from build123d import *

# Parameters (mm, degrees)
SKETCH1_W               = 292
SKETCH1_H               = 117
SKETCH1_R               = 1.75
BOSS_EXTRUDE1_DEPTH     = 4.5
SKETCH1_3_R             = 1.75
CUT_EXTRUDE1_DEPTH      = 4.5
MIRROR3_COPY_1_SKETCH_R = 1.75
MIRROR3_COPY_1_DEPTH    = 4.5
SKETCH2_W               = 35
SKETCH2_H               = 140
BOSS_EXTRUDE2_DEPTH     = 30
CHAMFER1_SIZE           = 10
CHAMFER1_SIZE2          = 15
CHAMFER2_SIZE           = 15
CHAMFER2_SIZE2          = 10


with BuildPart() as part:
    # Sketch1 → Boss-Extrude1 (new body)
    with BuildSketch(Plane.XY):
        Rectangle(SKETCH1_W, SKETCH1_H)
        with Locations((-90, 44)):
            Circle(SKETCH1_R, mode=Mode.SUBTRACT)
        with Locations((-90, 44)):
            Circle(SKETCH1_R)
    extrude(amount=BOSS_EXTRUDE1_DEPTH)

    # Sketch1_3 → Cut-Extrude1 (cut)
    with BuildSketch(Plane.XY):
        with Locations((-90, 44)):
            Circle(SKETCH1_3_R)
    cut_extrude1 = extrude(amount=CUT_EXTRUDE1_DEPTH, mode=Mode.SUBTRACT)

    # Mirror2: Cut-Extrude1 across plane
    add(cut_extrude1.mirror(Plane.ZX), mode=Mode.SUBTRACT)

    # Mirror3: Cut-Extrude1 across plane
    add(cut_extrude1.mirror(Plane(origin=(0, 0, 0), x_dir=(0, 0, 1), z_dir=(1, 0, 0))), mode=Mode.SUBTRACT)

    # Mirror3 copy 1 sketch → Mirror3 copy 1 (cut)
    with BuildSketch(Plane(origin=(0, 0, 0), x_dir=(-1, 0, 0), z_dir=(0, 0, 1))):
        with Locations((-90, 44)):
            Circle(MIRROR3_COPY_1_SKETCH_R)
    extrude(amount=MIRROR3_COPY_1_DEPTH, mode=Mode.SUBTRACT)

    # Sketch2 → Boss-Extrude2 (add)
    with BuildSketch(Plane(origin=(0, 0, 0), x_dir=(-1, 0, 0), z_dir=(0, 0, -1))):
        with Locations((-128.5, 11.5)):
            Rectangle(SKETCH2_W, SKETCH2_H)
    boss_extrude2 = extrude(amount=-BOSS_EXTRUDE2_DEPTH)

    # Chamfer1
    chamfer1_edges = [part.edges().sort_by_distance(p)[0] for p in [
        (128.5, 81.5, 0),
    ]]
    chamfer1_side = [part.faces().sort_by_distance(p)[0] for p in [
        (128.5, 81.5, 15),
    ]]
    chamfer(chamfer1_edges, length=CHAMFER1_SIZE, length2=CHAMFER1_SIZE2, reference=chamfer1_side[0])

    # Mirror5: Boss-Extrude2 across plane
    add(boss_extrude2.mirror(Plane(origin=(0, 0, 0), x_dir=(0, 0, 1), z_dir=(1, 0, 0))))

    # Chamfer2
    chamfer2_edges = [part.edges().sort_by_distance(p)[0] for p in [
        (-128.5, 81.5, 0),
    ]]
    chamfer2_side = [part.faces().sort_by_distance(p)[0] for p in [
        (-1.915975925, 2.0973848, 0),
    ]]
    chamfer(chamfer2_edges, length=CHAMFER2_SIZE, length2=CHAMFER2_SIZE2, reference=chamfer2_side[0])


solid = part.part
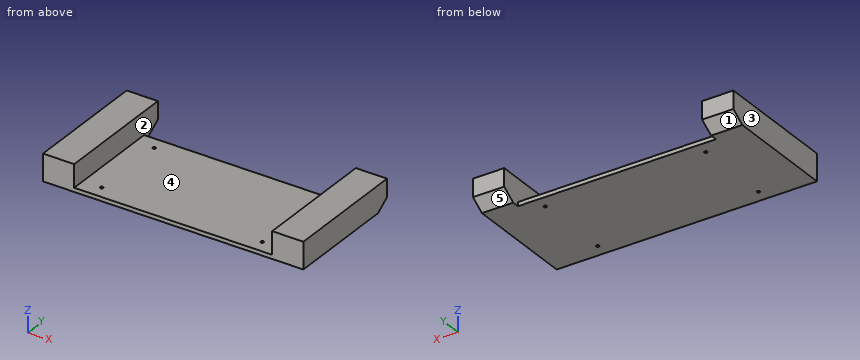
Geometry: final body of the model. Coordinates: model frame, mm. Face numbers are marked on the shaded views. A direction names the side the tool comes from. Coordinates: 2 decimals unless noted, no trailing zeros. Order: outer loops, then holes, each group sorted by start corner. A loop starts at its lowest first (then second) coordinate and runs counter-clockwise, first axis right, second up.
1) Section A-A (z = 24). Return loops of the section in (x, y), then the cut area to 3 significant figures.
Result sheet:
outline: (-146, -58.5) - (-111, -58.5) - (-111, 81.5) - (-146, 81.5) - close; (111, -58.5) - (146, -58.5) - (146, 81.5) - (111, 81.5) - close
area: 9,800 mm2
2) Section C-C (x = -6.5). Return loops of the section in (y, z), then the cut area to 4 significant figures.
Result sheet:
outline: (-58.5, 0) - (58.5, 0) - (58.5, 4.5) - (-58.5, 4.5) - close
area: 526.5 mm2
3) Section B-B (y = 21.5). Return loops of the section in (x, z), then the cut area to 3 significant figures.
Result sheet:
outline: (-146, 0) - (146, 0) - (146, 30) - (111, 30) - (111, 4.5) - (-111, 4.5) - (-111, 30) - (-146, 30) - close
area: 3,100 mm2
4) Draft query along X for the marked faces 1, 2 and 3. Return one class per face: released by +X, released by -X, zero draft, split by the parting line, or undercut.
Result sheet:
face 1: zero draft
face 2: undercut
face 3: released by -X
5) Set-up query: the marked faces 4 and 5. Return all of +Z, -Z, +X, -X, +Y, -Y with unobstructed straight access to the full face (end or side cutting, diameter ignored); none if empty.
Result sheet:
face 4: +Z, +Y, -Y
face 5: -Z, +X, -X, +Y
6) Ray query, probe 1 along Y at (x, z) = (90, 1.6); probe 2 along X at (y, z) = (-44, 2.25); probe 3 along X at (y, z) = (-33, 10). Return the intervals inside material, ascending.
Result sheet:
probe 1: y = -58.5 to -45.75, -42.25 to 42.25, 45.75 to 58.5
probe 2: x = -146 to -91.75, -88.25 to 88.25, 91.75 to 146
probe 3: x = -146 to -111, 111 to 146
7) First-contact query: P1, Ø3, axis at x = 90, y = 44, coming from the +Z side; P2, Ø4, axis at x = 7, y = 25.5, coming from the +Z side; P3, Ø5, axis at x = -44, z = 2.5, coming from the +Y side. Flat tips, straight axial feed; report the tip coordinate or a pass-through.
Result sheet:
P1: passes through
P2: stops at z = 4.5
P3: stops at y = 58.5
